from build123d import *

# Parameters (mm, degrees)
F0_W     = 21.674182
F0_H     = 15.005204
F1_DEPTH = 25
F2_DEPTH = 100


with BuildPart() as f1:
    # F0 (on Front) → F1 (new body)
    with BuildSketch(Plane.XZ):
        Polygon((58.353573, 27.231669), (-15.283082, 27.231669), (-15.283082, 12.226465), (-36.957264, 12.226465), (-36.957264, -36.679387), (58.353573, -36.679387), align=None)
        with Locations((-26.120173, 19.729067)):
            Rectangle(F0_W, F0_H)
    extrude(amount=F1_DEPTH)

    # F0 (on Front) → F2 (join)
    with BuildSketch(Plane.XZ):
        Polygon((-36.957264, 12.226465), (-36.957264, 27.231669), (-15.283082, 27.231669), (-15.283082, 44.181995), (-51.128846, 44.181995), (-51.128846, 12.226465), align=None)
    extrude(amount=F2_DEPTH)


solid = f1.part
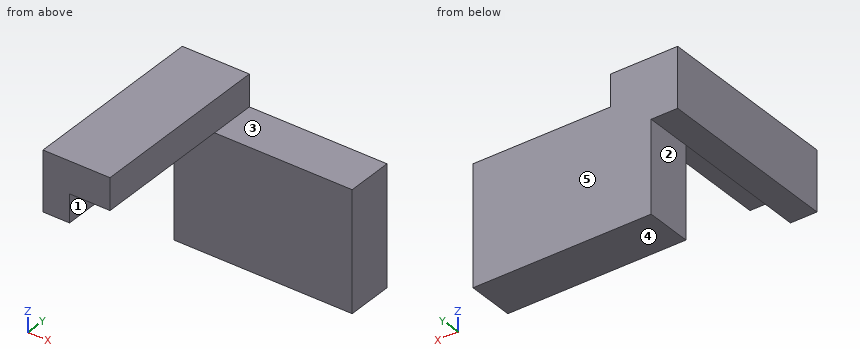
Can you work these out from the model? Positions are in its coordinate system, mm. Face numbers are marked on the shaded views. A direction names the side the tool comes from. Coordinates: 2 decimals unless noted, no trailing zeros. Order: outer loops, then holes, each group sorted by start corner. A loop starts at its lowest first (then second) coordinate and runs counter-clockwise, first axis right, second up. Notation, with made-up numbers: (-23, -21.5) - (27, -21.5) arc R25 cw to (27, -3.5) - close; hole circle Ø4 at (74.5, 20.25). An arc over 180 degrees is marked (long way). Answer as a JSON object with one key per item and string values. Group by question number.
Q1. I need wall thicknesses on line 1 (Z direction, x = -20.5, y = -31); line 2 (X direction, y = -6.5, z = -27.5); line 3 (X direction, y = -84.5, z = 21.5). Which ranges of each line are inside material? Lowest first, please. Write a range as from..to.
Q2. On a 3-axis mill with a long thin cutter (end or side, diameter ignored), from which of +Z, -Z, +X, -X, +Y, -Y can I reach the whole of each face in a straight line? I mean the marked faces 1, 2, 3, 4 and 5. Say none if no direction works.
Q3. Imagine slicing it at C-C (z = 19.5). Please give me the cut outline in (x, y), and give its area (3 significant figures).
Q4. Imagine slicing it at D-D (z = -13). Please give me the cut outline in (x, y).
Q5. Will these pins go through, and if not, where does the flat tip stop? P1, Ø7.5, axis at x = 9.5, y = -17.5, coming from the +Z side; P2, Ø15.5, axis at x = -43.5, y = -55, coming from the -Z side; P3, Ø19, axis at x = 23.5, z = 6, coming from the -Y side.
Q6. Imagine slicing it at B-B (x = -28). Please give me the cut outline in (y, z).
Q7. Imagine slicing it at A-A (y = -22.5). Please give me the cut outline in (x, z).
Determined:
{
 "1": {"line 1": "z = 27.23..44.18", "line 2": "x = -36.96..58.35", "line 3": "x = -51.13..-36.96"},
 "2": {"face 1": "-Z, +X, -Y", "face 2": "-Z, -X, +Y, -Y", "face 3": "+Z, +X, +Y, -Y", "face 4": "-Z, +X, -X, +Y, -Y", "face 5": "+Z, -Z, +X, -X, +Y"},
 "3": {"outline": "(-51.13, -100) - (-36.96, -100) - (-36.96, -25) - (58.35, -25) - (58.35, 0) - (-51.13, 0) - close", "area": "3,800 mm2"},
 "4": {"outline": "(-36.96, -25) - (58.35, -25) - (58.35, 0) - (-36.96, 0) - close"},
 "5": {"P1": "stops at z = 27.23", "P2": "stops at z = 12.23", "P3": "stops at y = -25"},
 "6": {"outline": "(-100, 27.23) - (-25, 27.23) - (-25, -36.68) - (0, -36.68) - (0, 44.18) - (-100, 44.18) - close"},
 "7": {"outline": "(-51.13, 12.23) - (-36.96, 12.23) - (-36.96, -36.68) - (58.35, -36.68) - (58.35, 27.23) - (-15.28, 27.23) - (-15.28, 44.18) - (-51.13, 44.18) - close"}
}
